Geometry: final body of the model. Coordinates: model frame, mm. A direction names the side the tool comes from. Round coordinates to 2 decimals unless told otherwise and drop trailing zeros. Write each loop counter-clockwise with the first axis right and the second up, starting at its lowest first coordinate (ties: lowest second). Pieces come first, ordered by that corner, then holes. Notation, with made-up numbers: M 19.25,33.5 L 33.25,33.5 A22 ccw 33.25,72.5 Z; hole C 82.5,40.5 d3. An arc over 180 degrees is marked long. Answer as CSV lines item,"result". Start each with the question number.
Q1. Section query D-D on x = -9.5. Output: boundary loops of the cut face in (y, z).
Q2. First-contact query: pin 1 (6 mm diameter, centred on x = -21.5, y = 14.5, fed in from +Z); pin 2 (2 mm diameter, centred on x = 0, y = 29.71, fed in from +Z); pin 3 (8.5 mm diameter, centred on x = -0.5, y = 5, fed in from +Z); pin 4 (3.5 mm diameter, centred on x = 0.22, y = -8.5, fed in from -Z). Flat tips, straight axial feed; report the tip coordinate or a pass-through.
Q3. Ray query, probe 1 along Y at (x, z) = (0, 2); probe 2 along Y at (x, z) = (0, 92); probe 3 along Y at (x, z) = (-0.5, 46.5) (3 decimals). Return the intervals inside material, ascending.
Q4. Section query B-B on x = 0. Give the number of separate pieces and of enclosed holes in the cut face, and give its area (3 significant figures).
Q5. Reachability of faces 1 (the cylindrical face through (-0.61, 11.47, 92.26)), 2 (the cylindrical face through (-22.89, -7.21, 44.37)), 3 (the cylindrical face through (0.01, -6.91, 90.74)) from +Z, -Z, +X, -X, +Y, -Y: full face, straight path, thin tool, end or side. Return the list, or none.
Q6. Section query A-A on z = 28. Output: boundary loops of the cut face in (x, y), and give its area (3 significant figures).
Q7. Mould query, pull axis Y, two halves, no side actions, for faces 4 (the flat face through (27, 0, 4)), 5 (the cylindrical face through (-0.569, 6.935, 90.74)), 6 (the cylindrical face through (-1.08, -4.88, 91.48)), 7 (the cylindrical face through (-0.081, 33.398, 1.972)). Classes: pulls with the +Y half, pulls with the -Y half, needs draft (parallel to the pull), parting line crosses it, or undercut.
```python
from build123d import *

# Parameters (mm, degrees)
SKETCH1_R           = 25
SKETCH1_R_2         = 24
BOSS_EXTRUDE1_DEPTH = 90
SKETCH2_R           = 25
SKETCH2_R_2         = 5
SKETCH2_R_3         = 1.6
BOSS_EXTRUDE2_DEPTH = 3
SKETCH3_R           = 3
CUT_EXTRUDE1_DEPTH  = 1.5
SKETCH4_R           = 1.7
SKETCH4_R_2         = 24
BOSS_EXTRUDE3_DEPTH = 4
SKETCH5_R           = 25
SKETCH5_R_2         = 23.322104889
SKETCH5_R_3         = 15.538295327
SKETCH5_R_4         = 14.475167561
BOSS_EXTRUDE4_DEPTH = 3


with BuildPart() as part:
    # Sketch1 → Boss-Extrude1 (new body)
    with BuildSketch(Plane(origin=(0, 0, 0), x_dir=(0, 1, 0), z_dir=(0, 0, 1))):
        with Locations(Location((0, 0, 0), (0, 0, 90))):
            Circle(SKETCH1_R)
        with Locations(Location((0, 0, 0), (0, 0, 90))):
            Circle(SKETCH1_R_2, mode=Mode.SUBTRACT)
    extrude(amount=BOSS_EXTRUDE1_DEPTH)

    # Sketch2 → Boss-Extrude2 (add)
    with BuildSketch(Plane(origin=(90, 0, 90), x_dir=(0, 1, 0), z_dir=(0, 0, 1))):
        with Locations(Location((0, 90, 0), (0, 0, 90))):
            Circle(SKETCH2_R)
        with Locations(Location((0, 90, 0), (0, 0, 270))):
            Circle(SKETCH2_R_2, mode=Mode.SUBTRACT)
        with Locations(Location((-8.497096587, 89.777852327, 0), (0, 0, 270))):
            Circle(SKETCH2_R_3, mode=Mode.SUBTRACT)
        with Locations(Location((8.497096587, 90.222147673, 0), (0, 0, 270))):
            Circle(SKETCH2_R_3, mode=Mode.SUBTRACT)
    extrude(amount=BOSS_EXTRUDE2_DEPTH)

    # Sketch3 → Cut-Extrude1 (cut)
    with BuildSketch(Plane.XY.offset(93)):
        with Locations((-0.222147673, 8.497096587)):
            Circle(SKETCH3_R)
        with Locations((0.222147673, -8.497096587)):
            Circle(SKETCH3_R)
    extrude(amount=-CUT_EXTRUDE1_DEPTH, mode=Mode.SUBTRACT)

    # Sketch4 → Boss-Extrude3 (add)
    with BuildSketch(Plane(origin=(0, 0, 0), x_dir=(1, 0, 0), z_dir=(0, 0, -1))):
        with BuildLine():
            ThreePointArc((-8.088357722, 23.655410995), (-17.67766953, 17.67766953), (-23.655410995, 8.088357722))
            ThreePointArc((-23.655410995, 8.088357722), (-25.999890745, 4.92208801), (-29.742595978, 3.6916382))
            ThreePointArc((-29.742595978, 3.6916382), (-33.398500606, 0), (-29.742595978, -3.6916382))
            ThreePointArc((-29.742595978, -3.6916382), (-25.999890745, -4.92208801), (-23.655410995, -8.088357722))
            ThreePointArc((-23.655410995, -8.088357722), (-17.67766953, -17.67766953), (-8.088357722, -23.655410995))
            ThreePointArc((-8.088357722, -23.655410995), (-4.92208801, -25.999890745), (-3.6916382, -29.742595978))
            ThreePointArc((-3.6916382, -29.742595978), (0, -33.398500606), (3.6916382, -29.742595978))
            ThreePointArc((3.6916382, -29.742595978), (4.92208801, -25.999890745), (8.088357722, -23.655410995))
            ThreePointArc((8.088357722, -23.655410995), (17.67766953, -17.67766953), (23.655410995, -8.088357722))
            ThreePointArc((23.655410995, -8.088357722), (25.999890745, -4.92208801), (29.742595978, -3.6916382))
            ThreePointArc((29.742595978, -3.6916382), (33.398500606, 0), (29.742595978, 3.6916382))
            ThreePointArc((29.742595978, 3.6916382), (25.999890745, 4.92208801), (23.655410995, 8.088357722))
            ThreePointArc((23.655410995, 8.088357722), (17.67766953, 17.67766953), (8.088357722, 23.655410995))
            ThreePointArc((8.088357722, 23.655410995), (4.92208801, 25.999890745), (3.6916382, 29.742595978))
            ThreePointArc((3.6916382, 29.742595978), (0, 33.398500606), (-3.6916382, 29.742595978))
            ThreePointArc((-3.6916382, 29.742595978), (-4.92208801, 25.999890745), (-8.088357722, 23.655410995))
        make_face()
        with Locations(Location((0, 29.706687772, 0), (0, 0, 180))):
            Circle(SKETCH4_R, mode=Mode.SUBTRACT)
        with Locations(Location((29.706687772, 0, 0), (0, 0, 180))):
            Circle(SKETCH4_R, mode=Mode.SUBTRACT)
        with Locations(Location((0, -29.706687772, 0), (0, 0, 180))):
            Circle(SKETCH4_R, mode=Mode.SUBTRACT)
        with Locations(Location((-29.706687772, 0, 0), (0, 0, 180))):
            Circle(SKETCH4_R, mode=Mode.SUBTRACT)
        with Locations(Location((0, 0, 0), (0, 0, 180))):
            Circle(SKETCH4_R_2, mode=Mode.SUBTRACT)
    extrude(amount=-BOSS_EXTRUDE3_DEPTH)

    # Sketch5 → Boss-Extrude4 (add)
    # profile 1 of 2: a face of its own
    with BuildSketch(Plane.XY.offset(93)):
        with Locations(Location((0, 0, 0), (0, 0, 161.123199836))):
            Circle(SKETCH5_R)
        Circle(SKETCH5_R_2, mode=Mode.SUBTRACT)
    # profile 2 of 2: a face of its own
    with BuildSketch(Plane.XY.offset(93)):
        Circle(SKETCH5_R_3)
        Circle(SKETCH5_R_4, mode=Mode.SUBTRACT)
    extrude(amount=BOSS_EXTRUDE4_DEPTH)


solid = part.part
```
Entries:
1,outline,"M -23.12,0 L -22.04,0 L -22.04,90 L 22.04,90 L 22.04,0 L 23.12,0 L 23.12,96 L 21.3,96 L 21.3,93 L 12.3,93 L 12.3,96 L 10.92,96 L 10.92,93 L -10.92,93 L -10.92,96 L -12.3,96 L -12.3,93 L -21.3,93 L -21.3,96 L -23.12,96 Z"
2,pin 1,"stops at z = 96"
2,pin 2,"passes through"
2,pin 3,"stops at z = 93"
2,pin 4,"stops at z = 90"
3,probe 1,"y = -33.4 to -31.41, -28.01 to -24, 24 to 28.01, 31.41 to 33.4"
3,probe 2,"y = -25 to -11.49, -5.51 to -5, 5 to 5.51, 11.49 to 25"
3,probe 3,"y = -24.995 to -23.995, 23.995 to 24.995"
4,separate pieces,"6"
4,enclosed holes,"0"
4,area,"329 mm^2"
5,face 1,"+Z"
5,face 2,"-Z"
5,face 3,"+Z, -Z"
6,outline,"C 0,0 d50; hole C 0,0 d48"
6,area,"154 mm^2"
7,face 4,"needs draft"
7,face 5,"undercut"
7,face 6,"undercut"
7,face 7,"pulls with the +Y half"
